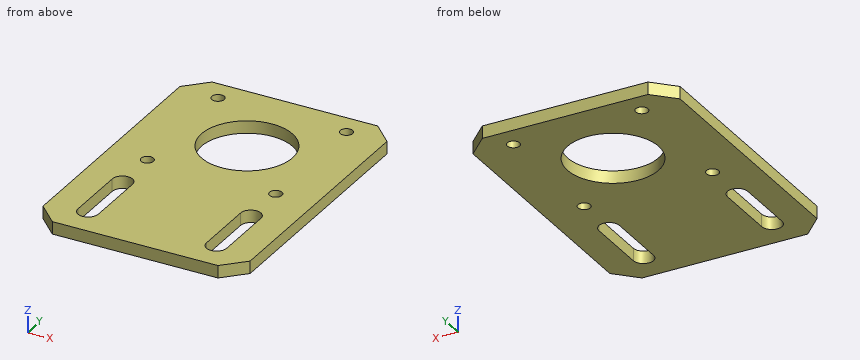
```python
from build123d import *

# Parameters (mm, degrees)
SKETCH1_R           = 11
SKETCH1_R_2         = 1.5
BOSS_EXTRUDE1_DEPTH = 3


with BuildPart() as part:
    # Sketch1 → Boss-Extrude1 (new body)
    with BuildSketch(Plane.XY):
        Polygon((20, -49), (-20, -49), (-25, -44), (-25, 16), (-20, 21), (20, 21), (25, 16), (25, -44), align=None)
        Circle(SKETCH1_R, mode=Mode.SUBTRACT)
        with Locations((-15.5, 15.5)):
            Circle(SKETCH1_R_2, mode=Mode.SUBTRACT)
        with Locations((15.5, 15.5)):
            Circle(SKETCH1_R_2, mode=Mode.SUBTRACT)
        with Locations((-15.5, -15.5)):
            Circle(SKETCH1_R_2, mode=Mode.SUBTRACT)
        with Locations((15.5, -15.5)):
            Circle(SKETCH1_R_2, mode=Mode.SUBTRACT)
        with BuildLine():
            Line((-13.05, -26.45), (-13.05, -41.45))
            ThreePointArc((-13.05, -41.45), (-15.5, -43.9), (-17.95, -41.45))
            Line((-17.95, -41.45), (-17.95, -26.45))
            ThreePointArc((-17.95, -26.45), (-15.5, -24), (-13.05, -26.45))
        make_face(mode=Mode.SUBTRACT)
        with BuildLine():
            Line((13.05, -26.45), (13.05, -41.45))
            ThreePointArc((13.05, -41.45), (15.5, -43.9), (17.95, -41.45))
            Line((17.95, -41.45), (17.95, -26.45))
            ThreePointArc((17.95, -26.45), (15.5, -24), (13.05, -26.45))
        make_face(mode=Mode.SUBTRACT)
    extrude(amount=BOSS_EXTRUDE1_DEPTH)


solid = part.part
```
The model under review builds one solid part; all positions refer to its coordinate system, in mm. Round coordinates to 2 decimals unless told otherwise and drop trailing zeros. Order: outer loops, then holes, each group sorted by start corner. A loop starts at its lowest first (then second) coordinate and runs counter-clockwise, first axis right, second up. Notation, with made-up numbers: M -23.5,10.5 L 28.5,10.5 A22 ccw 28.5,23.5 Z; hole C -21.75,26 d7. An arc over 180 degrees is marked long. Use a Markdown table: item, result.
1) Consider section B-B (x = -15.5). Write out the cut boundary in (y, z), then the cut area to 3 significant figures.
Report:
| item | result |
|---|---|
| outline | M -49,0 L -43.9,0 L -43.9,3 L -49,3 Z; M -24,0 L -17,0 L -17,3 L -24,3 Z; M -14,0 L 14,0 L 14,3 L -14,3 Z; M 17,0 L 21,0 L 21,3 L 17,3 Z |
| area | 132 mm^2 |
2) Consider section D-D (x = 0). Write out the cut boundary in (y, z).
Report:
| item | result |
|---|---|
| outline | M -49,0 L -11,0 L -11,3 L -49,3 Z; M 11,0 L 21,0 L 21,3 L 11,3 Z |
3) Wall thickness on line 1 along Y through (x, z) = (15.5, 1.15); line 2 along X through (y, z) = (-38.5, 1.55); line 3 along X through (y, z) = (-24.5, 1.6): over which ranges is each line inside the solid? List them lowest first. Write a range as [from, to].
Report:
| item | result |
|---|---|
| line 1 | [-49, -43.9], [-24, -17], [-14, 14], [17, 21] |
| line 2 | [-25, -17.95], [-13.05, 13.05], [17.95, 25] |
| line 3 | [-25, -16.98], [-14.02, 14.02], [16.98, 25] |
4) Consider section C-C (y = 0). Write out the cut boundary in (x, z).
Report:
| item | result |
|---|---|
| outline | M -25,0 L -11,0 L -11,3 L -25,3 Z; M 11,0 L 25,0 L 25,3 L 11,3 Z |
5) Consider section A-A (z = 0.95). Write out the cut boundary in (x, y).
Report:
| item | result |
|---|---|
| outline | M -25,-44 L -20,-49 L 20,-49 L 25,-44 L 25,16 L 20,21 L -20,21 L -25,16 Z; hole M -17.95,-41.45 A2.45 ccw -13.05,-41.45 L -13.05,-26.45 A2.45 ccw -17.95,-26.45 Z; hole C -15.5,-15.5 d3; hole C -15.5,15.5 d3; hole C 0,0 d22; hole M 13.05,-41.45 A2.45 ccw 17.95,-41.45 L 17.95,-26.45 A2.45 ccw 13.05,-26.45 Z; hole C 15.5,-15.5 d3; hole C 15.5,15.5 d3 |
